```python
from build123d import *

# Parameters (mm, degrees)
SKETCH1_W           = 70
SKETCH1_H           = 70
BOSS_EXTRUDE1_DEPTH = 35
SKETCH2_R           = 3.5
CUT_EXTRUDE1_DEPTH  = 71
SKETCH3_R           = 3.5
CUT_EXTRUDE2_DEPTH  = 71
SKETCH4_R           = 3.5
CUT_EXTRUDE3_DEPTH  = 71
CUT_EXTRUDE4_DEPTH  = 1


with BuildPart() as part:
    # Sketch1 → Boss-Extrude1 (new body, symmetric)
    with BuildSketch(Plane(origin=(0, 0, 0), x_dir=(1, 0, 0), z_dir=(0, 1, 0))):
        Rectangle(SKETCH1_W, SKETCH1_H)
    extrude(amount=BOSS_EXTRUDE1_DEPTH, both=True)

    # Sketch2 → Cut-Extrude1 (cut, through all)
    with BuildSketch(Plane(origin=(0, 35, 0), x_dir=(1, 0, 0), z_dir=(0, 1, 0))):
        Circle(SKETCH2_R)
    extrude(amount=-CUT_EXTRUDE1_DEPTH, mode=Mode.SUBTRACT)

    # Sketch3 → Cut-Extrude2 (cut, through all)
    with BuildSketch(Plane.XY.offset(35)):
        Circle(SKETCH3_R)
    extrude(amount=-CUT_EXTRUDE2_DEPTH, mode=Mode.SUBTRACT)

    # Sketch4 → Cut-Extrude3 (cut, through all)
    with BuildSketch(Plane(origin=(35, 0, 0), x_dir=(0, 0, -1), z_dir=(1, 0, 0))):
        Circle(SKETCH4_R)
    extrude(amount=-CUT_EXTRUDE3_DEPTH, mode=Mode.SUBTRACT)

    # Sketch5 → Cut-Extrude4 (cut)
    with BuildSketch(Plane.XZ.offset(35)):
        Polygon((7.303847577, -10.5), (7.303847577, -9), (12.5, -12), (7.303847577, -15), (7.303847577, -13.5), (-12.5, -13.5), (-12.5, -10.5), align=None)
    extrude(amount=-CUT_EXTRUDE4_DEPTH, mode=Mode.SUBTRACT)


solid = part.part
```
Here's how the part is built. I have some questions about the finished solid (model axes, mm). A direction names the side the tool comes from. Give positions to 0.01 mm unless a question says otherwise; leave off trailing zeros. Write each loop counter-clockwise with the first axis right and the second up, starting at its lowest first coordinate (ties: lowest second). Pieces come first, ordered by that corner, then holes. Notation, with made-up numbers: M 44,0 L 91,0 A27 ccw 91,39 Z; hole C -32.75,-16 d8. An arc over 180 degrees is marked long. Put each result on its own line as item: value. Start each with the question number.
Item 1: If we section it at B-B, the plane x = 0: Write out the boundary of the cut face in (y, z).
Item 2: If we section it at A-A, the plane z = 0: Write out the boundary of the cut face in (x, y).
Item 3: I need wall thicknesses on L1, parallel to Y at x = 0, z = -16. Which ranges of the line are inside material? Lowest first, please. Write a range as from..to.
Item 4: On a 3-axis mill with a long thin cutter (end or side, diameter ignored), from which of +Z, -Z, +X, -X, +Y, -Y can I reach the whole of each face in a straight line? I mean faces 5 (the flat face through (9.9, -34.5, -13.5)), 6 (the flat face through (7, 0, -35)). Say none if no direction works.
Item 5: Will these pins go through, and if not, where does the flat tip stop? pin 1 (4 mm diameter, centred on x = 0, y = 0, fed in from +Z); pin 2 (1.8 mm diameter, centred on x = 0, z = -12.5, fed in from -Y).
Item 6: Thinking about a two-plate mould opening in Y: for faces 1 (the cylindrical face through (18.965, -1.341, -3.233)), 2 (the flat face through (7, 0, 35)), 3 (the cylindrical face through (3.233, -1.341, 18.965)), 4 (the flat face through (7, 35, 0)), which applies, +Y half, -Y half, draft (parallel to the pull), parting line (faces both ways), or undercut?
Values:
1. outline: M -35,-35 L -3.5,-35 L -3.5,-3.5 L -35,-3.5 L -35,-10.5 L -34,-10.5 L -34,-13.5 L -35,-13.5 Z; M -35,3.5 L -3.5,3.5 L -3.5,35 L -35,35 Z; M 3.5,-35 L 35,-35 L 35,-3.5 L 3.5,-3.5 Z; M 3.5,3.5 L 35,3.5 L 35,35 L 3.5,35 Z
2. outline: M -35,-35 L -3.5,-35 L -3.5,-3.5 L -35,-3.5 Z; M -35,3.5 L -3.5,3.5 L -3.5,35 L -35,35 Z; M 3.5,-35 L 35,-35 L 35,-3.5 L 3.5,-3.5 Z; M 3.5,3.5 L 35,3.5 L 35,35 L 3.5,35 Z
3. L1: -35..-3.5, 3.5..35
4. face 5: -Y
4. face 6: -Z, +X, -X, +Y, -Y
5. pin 1: through
5. pin 2: y = -34
6. face 1: undercut
6. face 2: draft
6. face 3: undercut
6. face 4: +Y half
